Build history of the part. All positions in model axes, mm. Give positions to 0.01 mm unless a question says otherwise; leave off trailing zeros. One line per question, with ' | ' between items. Start each with the question number.
(1) Slice it at A-A, the plane y = 2.7. Give the number of separate pieces and of enclosed holes in the cut face, then the cut area to 3 significant figures.
(2) Mould opens along X. For faces 1 (the face through (-5, 2, -46.089)), 2 (the face through (-88.88, 2.46, 18.02)), 3 (the face through (-103.911, 2, 5)) say: pulls with the +X half, pulls with the -X half, needs draft (parallel to the pull), parting line crosses it, or undercut.
(3) Flat gauge pins, fed straight in: pin 1 Ø9.5 at (x, z) = (33.59, 41.41) entering from -Y; pin 2 Ø5.5 at (x, z) = (8.59, -8.59) entering from +Y. Where does each tip first touch, or does it go through?
```python
from build123d import *

# Parameters (mm, degrees)
SKETCH_1_W      = 200
SKETCH_1_H      = 100
SKETCH_1_R      = 3
EXTRUDE_1_DEPTH = 5


with BuildPart() as part:
    # 草图1 → 凸台-拉伸1 (new body)
    with BuildSketch(Plane(origin=(0, 0, 0), x_dir=(1, 0, 0), z_dir=(0, 1, 0))):
        with Locations((-3.910614525, -3.910614525)):
            Rectangle(SKETCH_1_W, SKETCH_1_H)
        with Locations(Location((-91.410614525, -41.410614525, 0), (0, 0, 270))):
            Circle(SKETCH_1_R, mode=Mode.SUBTRACT)
        with Locations(Location((-66.410614525, -41.410614525, 0), (0, 0, 270))):
            Circle(SKETCH_1_R, mode=Mode.SUBTRACT)
        with Locations(Location((-41.410614525, -41.410614525, 0), (0, 0, 270))):
            Circle(SKETCH_1_R, mode=Mode.SUBTRACT)
        with Locations(Location((-16.410614525, -41.410614525, 0), (0, 0, 270))):
            Circle(SKETCH_1_R, mode=Mode.SUBTRACT)
        with Locations(Location((8.589385475, -41.410614525, 0), (0, 0, 270))):
            Circle(SKETCH_1_R, mode=Mode.SUBTRACT)
        with Locations(Location((33.589385475, -41.410614525, 0), (0, 0, 270))):
            Circle(SKETCH_1_R, mode=Mode.SUBTRACT)
        with Locations(Location((58.589385475, -41.410614525, 0), (0, 0, 270))):
            Circle(SKETCH_1_R, mode=Mode.SUBTRACT)
        with Locations(Location((83.589385475, -41.410614525, 0), (0, 0, 270))):
            Circle(SKETCH_1_R, mode=Mode.SUBTRACT)
        with Locations(Location((-66.410614525, -16.410614525, 0), (0, 0, 270))):
            Circle(SKETCH_1_R, mode=Mode.SUBTRACT)
        with Locations(Location((-41.410614525, -16.410614525, 0), (0, 0, 270))):
            Circle(SKETCH_1_R, mode=Mode.SUBTRACT)
        with Locations(Location((-16.410614525, -16.410614525, 0), (0, 0, 270))):
            Circle(SKETCH_1_R, mode=Mode.SUBTRACT)
        with Locations(Location((8.589385475, -16.410614525, 0), (0, 0, 270))):
            Circle(SKETCH_1_R, mode=Mode.SUBTRACT)
        with Locations(Location((33.589385475, -16.410614525, 0), (0, 0, 270))):
            Circle(SKETCH_1_R, mode=Mode.SUBTRACT)
        with Locations(Location((58.589385475, -16.410614525, 0), (0, 0, 270))):
            Circle(SKETCH_1_R, mode=Mode.SUBTRACT)
        with Locations(Location((83.589385475, -16.410614525, 0), (0, 0, 270))):
            Circle(SKETCH_1_R, mode=Mode.SUBTRACT)
        with Locations(Location((-66.410614525, 8.589385475, 0), (0, 0, 270))):
            Circle(SKETCH_1_R, mode=Mode.SUBTRACT)
        with Locations(Location((-41.410614525, 8.589385475, 0), (0, 0, 270))):
            Circle(SKETCH_1_R, mode=Mode.SUBTRACT)
        with Locations(Location((-16.410614525, 8.589385475, 0), (0, 0, 270))):
            Circle(SKETCH_1_R, mode=Mode.SUBTRACT)
        with Locations(Location((8.589385475, 8.589385475, 0), (0, 0, 270))):
            Circle(SKETCH_1_R, mode=Mode.SUBTRACT)
        with Locations(Location((33.589385475, 8.589385475, 0), (0, 0, 270))):
            Circle(SKETCH_1_R, mode=Mode.SUBTRACT)
        with Locations(Location((58.589385475, 8.589385475, 0), (0, 0, 270))):
            Circle(SKETCH_1_R, mode=Mode.SUBTRACT)
        with Locations(Location((83.589385475, 8.589385475, 0), (0, 0, 270))):
            Circle(SKETCH_1_R, mode=Mode.SUBTRACT)
        with Locations(Location((-66.410614525, 33.589385475, 0), (0, 0, 270))):
            Circle(SKETCH_1_R, mode=Mode.SUBTRACT)
        with Locations(Location((-41.410614525, 33.589385475, 0), (0, 0, 270))):
            Circle(SKETCH_1_R, mode=Mode.SUBTRACT)
        with Locations(Location((-16.410614525, 33.589385475, 0), (0, 0, 270))):
            Circle(SKETCH_1_R, mode=Mode.SUBTRACT)
        with Locations(Location((8.589385475, 33.589385475, 0), (0, 0, 270))):
            Circle(SKETCH_1_R, mode=Mode.SUBTRACT)
        with Locations(Location((33.589385475, 33.589385475, 0), (0, 0, 270))):
            Circle(SKETCH_1_R, mode=Mode.SUBTRACT)
        with Locations(Location((58.589385475, 33.589385475, 0), (0, 0, 270))):
            Circle(SKETCH_1_R, mode=Mode.SUBTRACT)
        with Locations(Location((83.589385475, 33.589385475, 0), (0, 0, 270))):
            Circle(SKETCH_1_R, mode=Mode.SUBTRACT)
        with Locations(Location((-91.410614525, -16.410614525, 0), (0, 0, 270))):
            Circle(SKETCH_1_R, mode=Mode.SUBTRACT)
        with Locations(Location((-91.410614525, 8.589385475, 0), (0, 0, 270))):
            Circle(SKETCH_1_R, mode=Mode.SUBTRACT)
        with Locations(Location((-91.410614525, 33.589385475, 0), (0, 0, 270))):
            Circle(SKETCH_1_R, mode=Mode.SUBTRACT)
    extrude(amount=EXTRUDE_1_DEPTH)


solid = part.part
```
Final values:
1) separate pieces: 1 | enclosed holes: 32 | area: 19,100 mm2
2) face 1: needs draft | face 2: undercut | face 3: pulls with the -X half
3) pin 1: y = 0 | pin 2: through
